from build123d import *

# Parameters (mm, degrees)
SKETCH1_W           = 21.717
SKETCH1_H           = 47.117
BOSS_EXTRUDE1_DEPTH = 0.762
SKETCH2_W           = 25.4
SKETCH2_H           = 50.8
BOSS_EXTRUDE2_DEPTH = 3.175
SKETCH3_R           = 2.5527
CUT_EXTRUDE1_DEPTH  = 4.937
FILLET1_R           = 2.54
FILLET3_R           = 0.79375


with BuildPart() as part:
    # Sketch1 → Boss-Extrude1 (new body)
    with BuildSketch(Plane(origin=(0, 0, 0), x_dir=(1, 0, 0), z_dir=(0, 1, 0))):
        Rectangle(SKETCH1_W, SKETCH1_H)
    extrude(amount=BOSS_EXTRUDE1_DEPTH)

    # Sketch2 → Boss-Extrude2 (add)
    with BuildSketch(Plane(origin=(0, 0.762, 0), x_dir=(1, 0, 0), z_dir=(0, 1, 0))):
        Rectangle(SKETCH2_W, SKETCH2_H)
    extrude(amount=BOSS_EXTRUDE2_DEPTH)

    # Sketch3 → Cut-Extrude1 (cut, through all)
    with BuildSketch(Plane(origin=(0, 3.937, 0), x_dir=(1, 0, 0), z_dir=(0, 1, 0))):
        with Locations((0, 12.7)):
            Circle(SKETCH3_R)
        with Locations((0, -12.7)):
            Circle(SKETCH3_R)
    extrude(amount=-CUT_EXTRUDE1_DEPTH, mode=Mode.SUBTRACT)

    # Fillet1
    fillet1_edges = [part.edges().sort_by_distance(p)[0] for p in [
        (12.7, 2.3495, 25.4),
        (12.7, 2.3495, -25.4),
        (-12.7, 2.3495, -25.4),
        (-12.7, 2.3495, 25.4),
        (-10.8585, 0.381, -23.5585),
        (10.8585, 0.381, -23.5585),
        (10.8585, 0.381, 23.5585),
        (-10.8585, 0.381, 23.5585),
    ]]
    fillet(fillet1_edges, radius=FILLET1_R)

    # Fillet3
    fillet3_edges = [part.edges().sort_by_distance(p)[0] for p in [
        (0, 3.937, -25.4),
        (12.7, 3.937, 0),
        (-12.7, 3.937, 0),
        (0, 3.937, 25.4),
        (-11.956051224, 3.937, 24.656051224),
        (-11.956051224, 3.937, -24.656051224),
        (11.956051224, 3.937, 24.656051224),
        (11.956051224, 3.937, -24.656051224),
    ]]
    fillet(fillet3_edges, radius=FILLET3_R)


solid = part.part
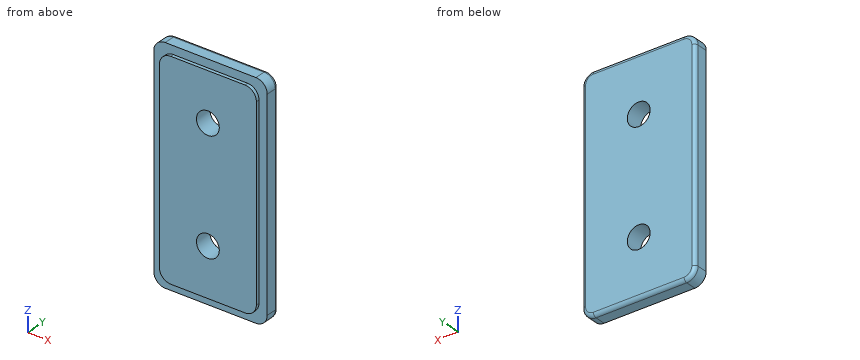
Geometry: final body of the model. Coordinates: model frame, mm. Coordinates: 2 decimals unless noted, no trailing zeros. Order: outer loops, then holes, each group sorted by start corner. A loop starts at its lowest first (then second) coordinate and runs counter-clockwise, first axis right, second up.
1) Section B-B (y = 2.1). Return loops of the section in (x, z), then the cut area to 3 significant figures.
Result sheet:
outline: (-12.7, -22.86) arc R2.54 ccw to (-10.16, -25.4) - (10.16, -25.4) arc R2.54 ccw to (12.7, -22.86) - (12.7, 22.86) arc R2.54 ccw to (10.16, 25.4) - (-10.16, 25.4) arc R2.54 ccw to (-12.7, 22.86) - close; hole circle Ø5.11 at (0, -12.7); hole circle Ø5.11 at (0, 12.7)
area: 1,240 mm2
2) Ray query, probe 1 along Z at (x, y) = (0, 1.45); probe 2 along X at (y, z) = (1.75, -12.7); probe 3 along Z at (x, y) = (1, 0.3). Return the intervals inside material, ascending.
Result sheet:
probe 1: z = -25.4 to -15.25, -10.15 to 10.15, 15.25 to 25.4
probe 2: x = -12.7 to -2.55, 2.55 to 12.7
probe 3: z = -23.56 to -15.05, -10.35 to 10.35, 15.05 to 23.56
3) First-contact query: P1, Ø12, axis at x = 9, z = -0.5, coming from the -Y side; P2, Ø4, axis at x = 0, z = -12.7, coming from the -Y side. Flat tips, straight axial feed; report the tip coordinate or a pass-through.
Result sheet:
P1: stops at y = 0
P2: passes through
4) Section D-D (x = 7.5). Return loops of the section in (y, z).
Result sheet:
outline: (0, -23.56) - (0.76, -23.56) - (0.76, -25.4) - (3.14, -25.4) arc R0.79 ccw to (3.94, -24.61) - (3.94, 24.61) arc R0.79 ccw to (3.14, 25.4) - (0.76, 25.4) - (0.76, 23.56) - (0, 23.56) - close
5) Section C-C (x = 0). Return loops of the section in (y, z).
Result sheet:
outline: (0, -23.56) - (0.76, -23.56) - (0.76, -25.4) - (3.14, -25.4) arc R0.79 ccw to (3.94, -24.61) - (3.94, -15.25) - (0, -15.25) - close; (0, -10.15) - (3.94, -10.15) - (3.94, 10.15) - (0, 10.15) - close; (0, 15.25) - (3.94, 15.25) - (3.94, 24.61) arc R0.79 ccw to (3.14, 25.4) - (0.76, 25.4) - (0.76, 23.56) - (0, 23.56) - close
6) Section A-A (z = 12.7). Return loops of the section in (x, y).
Result sheet:
outline: (-12.7, 0.76) - (-10.86, 0.76) - (-10.86, 0) - (-2.55, 0) - (-2.55, 3.94) - (-11.91, 3.94) arc R0.79 ccw to (-12.7, 3.14) - close; (2.55, 0) - (10.86, 0) - (10.86, 0.76) - (12.7, 0.76) - (12.7, 3.14) arc R0.79 ccw to (11.91, 3.94) - (2.55, 3.94) - close
